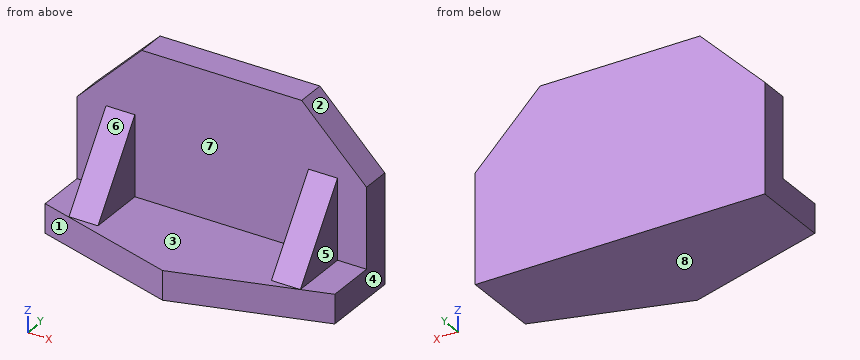
from build123d import *

# Parameters (mm, degrees)
F0_W      = 127
F0_H      = 76.2
F1_DEPTH  = 53.848
F2_W      = 127
F2_H      = 41.148
F3_DEPTH  = 63.5
F5_DEPTH  = 12.7
F7_DEPTH  = 12.7
F8_W      = 12.7
F8_H      = 26.142063
F9_DEPTH  = 35.052
F11_DEPTH = 12.7
F12_W     = 12.7
F12_H     = 25.67689
F13_DEPTH = 35.052
F15_DEPTH = 12.7


with BuildPart() as f1:
    # F0 (on Front) → F1 (new body)
    with BuildSketch(Plane.XZ):
        with Locations((-1.86439, -12.836598)):
            Rectangle(F0_W, F0_H)
    extrude(amount=F1_DEPTH)

    # F2 (on face) → F3 (cut)
    with BuildSketch(Plane.XY.offset(25.263402)):
        with Locations((-1.86439, -33.274)):
            Rectangle(F2_W, F2_H)
    extrude(amount=-F3_DEPTH, mode=Mode.SUBTRACT)

    # F4 (on face) → F5 (cut)
    with BuildSketch(Plane.XZ.offset(12.7)):
        Polygon((-36.91639, 25.263402), (-65.36439, 25.263402), (-65.36439, -3.184598), align=None)
        Polygon((61.63561, 25.263402), (33.18761, 25.263402), (61.63561, -3.184598), align=None)
    extrude(amount=-F5_DEPTH, mode=Mode.SUBTRACT)

    # F6 (on face) → F7 (cut)
    with BuildSketch(Plane.XY.offset(-38.236598)):
        Polygon((-65.36439, -53.848), (-1.86439, -53.848), (-65.36439, -34.798), align=None)
        Polygon((-1.86439, -53.848), (61.63561, -53.848), (61.63561, -34.798), align=None)
    extrude(amount=-F7_DEPTH, mode=Mode.SUBTRACT)

    # F8 (on face) → F9 (join)
    with BuildSketch(Plane.XY.offset(-38.236598)):
        with Locations((42.58561, -25.771031)):
            Rectangle(F8_W, F8_H)
    extrude(amount=F9_DEPTH)

    # F10 (on face) → F11 (cut)
    with BuildSketch(Plane.YZ.offset(48.93561)):
        Polygon((-38.842063, -38.236598), (-38.608, -38.236598), (-12.7, -3.184598), (-38.842063, -3.184598), align=None)
    extrude(amount=-F11_DEPTH, mode=Mode.SUBTRACT)

    # F12 (on face) → F13 (join)
    with BuildSketch(Plane.XY.offset(-38.236598)):
        with Locations((-46.31439, -25.538445)):
            Rectangle(F12_W, F12_H)
    extrude(amount=F13_DEPTH)

    # F14 (on face) → F15 (cut)
    with BuildSketch(Plane(origin=(-52.66439, 0, 0), x_dir=(0, -1, 0), z_dir=(-1, 0, 0))):
        Polygon((38.37689, -3.184598), (12.7, -3.184598), (38.37689, -38.236598), align=None)
    extrude(amount=-F15_DEPTH, mode=Mode.SUBTRACT)


solid = f1.part
The listing builds one solid part. Answer for the finished solid, in the listing's coordinates (mm). Face numbers are marked on the shaded views. A direction names the side the tool comes from. Round coordinates to 2 decimals unless told otherwise and drop trailing zeros. Loops run counter-clockwise (first coordinate to the right, second up) from the corner with the lowest first, then second, coordinate; pieces in that order, holes last. Notation, with made-up numbers: M 52.5,-29.5 L 97.5,-29.5 A29 cw 97.5,-8.5 Z; hole C 63.25,-20.75 d5. An arc over 180 degrees is marked long. Write each question's results on one line, items separated by ' | '. Start each with the question number.
1) Which of the six approach directions +Z, -Z, +X, -X, +Y, -Y give full straight-line access (tool end or side, diameter ignored) to the marked faces 4, 5, 6, 7 and 8?
2) Straight lines are drawn through the part: probe 1 along X at (y, z) = (-20, -33.5); probe 2 along Y at (x, z) = (16, 9.5); probe 3 along Z at (x, y) = (14.5, -25). For each, find the intervals that lie inside material, in ascending order.
3) Find section A-A on z = -44.5. Write down the section's boundary in (x, y), plus the area to 3 significant figures.
4) Determine the mould class of the marked faces 1, 2 and 3 for opening direction X: pulls with the +X half, pulls with the -X half, needs draft (parallel to the pull), parting line crosses it, or undercut.
5) Find section B-B on y = -36.5. Write down the section's boundary in (x, z), plus the area to 3 significant figures.
6) Each of these flat-tipped pins is pushed along its axis until it touches: pin 1 (5 mm diameter, centred on x = 40, z = -4, fed in from -Y); pin 2 (2 mm diameter, centred on x = 10.5, z = -38.5, fed in from -Y); pin 3 (4 mm diameter, centred on x = 4.5, z = -1, fed in from +Y); pin 4 (13 mm diameter, centred on y = -21.5, z = -22.5, fed in from +X). Where does it stop, or does it pass through?
7) Find section C-C on x = 25. Write down the section's boundary in (y, z), plus the area to 3 significant figures.
8) Find section D-D on z = -15. Write down the section's boundary in (x, y), plus the area to 3 significant figures.
Final values:
1) face 4: +Z, -Z, +X, +Y, -Y | face 5: +Z, +X, -Y | face 6: +Z, -X, -Y | face 7: +Z, -Y | face 8: -Z, +X, -X, +Y, -Y
2) probe 1: -52.66 to -39.96, 36.24 to 48.94 | probe 2: -12.7 to 0 | probe 3: -50.94 to -38.24
3) outline: M -65.36,-34.8 L -1.86,-53.85 L 61.64,-34.8 L 61.64,0 L -65.36,0 Z | area: 5,630 mm²
4) face 1: pulls with the -X half | face 2: pulls with the +X half | face 3: undercut
5) outline: M -59.69,-50.94 L 55.96,-50.94 L 55.96,-38.24 L 48.94,-38.24 L 48.94,-35.38 L 36.24,-35.38 L 36.24,-38.24 L -39.96,-38.24 L -39.96,-35.67 L -52.66,-35.67 L -52.66,-38.24 L -59.69,-38.24 Z | area: 1,540 mm²
6) pin 1: y = -15.15 | pin 2: y = -50.44 | pin 3: y = 0 | pin 4: x = 48.94
7) outline: M -45.79,-50.94 L 0,-50.94 L 0,25.26 L -12.7,25.26 L -12.7,-38.24 L -45.79,-38.24 Z | area: 1,390 mm²
8) outline: M -65.36,-12.7 L -52.66,-12.7 L -52.66,-21.36 L -39.96,-21.36 L -39.96,-12.7 L 36.24,-12.7 L 36.24,-21.43 L 48.94,-21.43 L 48.94,-12.7 L 61.64,-12.7 L 61.64,0 L -65.36,0 Z | area: 1,830 mm²
